The listing builds one solid part. Answer for the finished solid, in the listing's coordinates (mm). Coordinates: 2 decimals unless noted, no trailing zeros. Order: outer loops, then holes, each group sorted by start corner. A loop starts at its lowest first (then second) coordinate and runs counter-clockwise, first axis right, second up. Notation, with made-up numbers: (85.5, 37) -> (95.5, 37) arc R7 cw to (95.5, 43) -> close; hole circle Ø4 at (5, -25.75). An arc over 180 degrees is marked (long way). Return JSON: item names as keys, results as strings.
from build123d import *

# Parameters (mm, degrees)
F0_R     = 18
F1_DEPTH = 16
F2_D     = 8


with BuildPart() as f1:
    # F0 (on Front) → F1 (new body)
    with BuildSketch(Plane.XZ):
        with BuildLine():
            Line((-39.285714, -9.035079), (-10.714286, -22.587698))
            ThreePointArc((-10.714286, -22.587698), (0, -25), (10.714286, -22.587698))
            Line((10.714286, -22.587698), (39.285714, -9.035079))
            ThreePointArc((39.285714, -9.035079), (45, 0), (39.285714, 9.035079))
            Line((39.285714, 9.035079), (10.714286, 22.587698))
            ThreePointArc((10.714286, 22.587698), (0, 25), (-10.714286, 22.587698))
            Line((-10.714286, 22.587698), (-39.285714, 9.035079))
            ThreePointArc((-39.285714, 9.035079), (-45, 0), (-39.285714, -9.035079))
        make_face()
        Circle(F0_R, mode=Mode.SUBTRACT)
    extrude(amount=F1_DEPTH)

    # F2 (through all)
    with Locations(Plane(origin=(0, 0, 0), x_dir=(1, 0, 0), z_dir=(0, 1, 0))):
        with Locations((35, 0), (-35, 0)):
            Hole(F2_D / 2)


solid = f1.part
1. The part is cut by section A-A on y = -2.5. Give the vertices of the cut face in (x, z).
Answer block:
{"outline": "(-39.29, -9.04) -> (-10.71, -22.59) arc R25 ccw to (10.71, -22.59) -> (39.29, -9.04) arc R10 ccw to (39.29, 9.04) -> (10.71, 22.59) arc R25 ccw to (-10.71, 22.59) -> (-39.29, 9.04) arc R10 ccw to start; hole circle Ø8 at (-35, 0); hole circle Ø36 at (0, 0); hole circle Ø8 at (35, 0)"}
2. The part is cut by section C-C on z = 0. Give the vertices of the cut face in (x, y).
Answer block:
{"outline": "(-45, -16) -> (-39, -16) -> (-39, 0) -> (-45, 0) -> close; (-31, -16) -> (-18, -16) -> (-18, 0) -> (-31, 0) -> close; (18, -16) -> (31, -16) -> (31, 0) -> (18, 0) -> close; (39, -16) -> (45, -16) -> (45, 0) -> (39, 0) -> close"}
3. Determine the mould class of faces 1 (the face through (9, -16, 17)), 2 (the face through (0, -8, 25)), 3 (the face through (-31.8, -8.1, 2.4)) for opening direction X: pulls with the +X half, pulls with the -X half, needs draft (parallel to the pull), parting line crosses it, or undercut.
Answer block:
{"face 1": "needs draft", "face 2": "parting line crosses it", "face 3": "undercut"}
4. Consider line 1 (Z direction, x = -35, y = -10.75); line 2 (X direction, y = -7.25, z = 12); line 3 (Z direction, x = 3.5, y = -11.75). Determine where each line is inside the solid, lowest interval first. Write a range as from..to.
Answer block:
{"line 1": "z = -11.07..-4, 4..11.07", "line 2": "x = -33.04..-13.42, 13.42..33.04", "line 3": "z = -24.75..-17.66, 17.66..24.75"}
5. Each of these flat-tipped pins is pushed along its axis until it touches: pin 1 Ø6 at (y, z) = (-6.5, 13) entering from +X; pin 2 Ø4 at (x, y) = (15.5, -7) entering from -Z; pin 3 Ø1 at (y, z) = (-2.5, 8.5) entering from +X; pin 4 Ø10 at (x, z) = (5, 9.5) entering from -Y. Where does it stop, or does it pass through?
Answer block:
{"pin 1": "stops at x = 37.25", "pin 2": "stops at z = -21.27", "pin 3": "stops at x = 41", "pin 4": "passes through"}
6. The part is cut by section D-D on z = 15. Give the vertices of the cut face in (x, y), and give its area (3 significant figures).
Answer block:
{"outline": "(-26.71, -16) -> (-9.95, -16) -> (-9.95, 0) -> (-26.71, 0) -> close; (9.95, -16) -> (26.71, -16) -> (26.71, 0) -> (9.95, 0) -> close", "area": "536 mm2"}
7. The part is cut by section B-B on x = 0. Give the vertices of the cut face in (y, z).
Answer block:
{"outline": "(-16, -25) -> (0, -25) -> (0, -18) -> (-16, -18) -> close; (-16, 18) -> (0, 18) -> (0, 25) -> (-16, 25) -> close"}
